```python
from build123d import *

# Parameters (mm, degrees)
BOSS_EXTRU_1_DEPTH      = 4
TROU_TARAUD_M42_D       = 3.3
TROU_TARAUD_M43_D       = 3.3
TROU_TARAUD_M43_DEPTH   = 15.5
TROU_TARAUD_M43_TIP     = 0.991420021
CONG_1_R                = 10
ENL_V_START             = -9
ENL_V_MAT_EXTRU_1_DEPTH = 10
CHANFREIN1_SIZE         = 1


with BuildPart() as part:
    # Esquisse1 → Boss.-Extru.1 (new body, symmetric)
    with BuildSketch(Plane.XY):
        with BuildLine():
            Line((-29, 0), (29, 0))
            Line((29, 0), (42.125962847, 19.175742472))
            ThreePointArc((42.125962847, 19.175742472), (42.080485732, 24.889573705), (36.705904774, 26.829629131))
            Line((36.705904774, 26.829629131), (0, 16.99431159))
            Line((0, 16.99431159), (-36.705904774, 26.829629131))
            ThreePointArc((-36.705904774, 26.829629131), (-42.080485732, 24.889573705), (-42.125962847, 19.175742472))
            Line((-42.125962847, 19.175742472), (-29, 0))
        make_face()
    extrude(amount=BOSS_EXTRU_1_DEPTH, both=True)

    # Trou taraudé M42 (through all)
    with Locations(Plane.XY.offset(4)):
        with Locations((-38, 22), (38, 22), (-33, 16), (33, 16)):
            Hole(TROU_TARAUD_M42_D / 2)

    # Trou taraudé M43
    with Locations(Plane(origin=(0, 0, 0), x_dir=(-1, 0, 0), z_dir=(0, -1, 0))):
        with Locations((20, 0), (-20, 0), (0, -0.5)):
            Hole(TROU_TARAUD_M43_D / 2, depth=TROU_TARAUD_M43_DEPTH)
            with Locations((0, 0, -(TROU_TARAUD_M43_DEPTH + TROU_TARAUD_M43_TIP / 2))):  # 118° drill point
                Cone(0, TROU_TARAUD_M43_D / 2, TROU_TARAUD_M43_TIP, mode=Mode.SUBTRACT)

    # Congé1
    cong_1_edges = [part.edges().sort_by_distance(p)[0] for p in [
        (0, 16.99431159, 0),
    ]]
    fillet(cong_1_edges, radius=CONG_1_R)

    # Esquisse8 → Enlèv. mat.-Extru.1 (cut)
    with BuildSketch(Plane.XY.offset(4).offset(ENL_V_START)):
        with BuildLine():
            Line((-3, 10.703460795), (-3, 10.5))
            ThreePointArc((-3, 10.5), (-3.732233047, 8.732233047), (-5.5, 8))
            Line((-5.5, 8), (-22.251200511, 8))
            ThreePointArc((-22.251200511, 8), (-23.417321879, 8.288629168), (-24.314181934, 9.087871236))
            Line((-24.314181934, 9.087871236), (-28.247222943, 14.833657842))
            ThreePointArc((-28.247222943, 14.833657842), (-28.224484386, 17.690573459), (-25.537193907, 18.660601172))
            Line((-25.537193907, 18.660601172), (-4.852952387, 13.118275361))
            ThreePointArc((-4.852952387, 13.118275361), (-3.516616649, 12.225364367), (-3, 10.703460795))
        make_face()
    enl_v_mat_extru_1 = extrude(amount=ENL_V_MAT_EXTRU_1_DEPTH, mode=Mode.SUBTRACT)

    # Symétrie1: Enlèv. mat.-Extru.1 across plane
    add(enl_v_mat_extru_1.mirror(Plane(origin=(0, 0, 0), x_dir=(0, 0, 1), z_dir=(1, 0, 0))), mode=Mode.SUBTRACT)

    # Chanfrein1
    chanfrein1_edges = [part.edges().sort_by_distance(p)[0] for p in [
        (-35.562981423, 9.587871236, -4),
        (-42.080485732, 24.889573705, 4),
        (-42.080485732, 24.889573705, -4),
        (-19.647047613, 22.258722131, -4),
        (-35.562981423, 9.587871236, 4),
        (35.562981423, 9.587871236, 4),
        (42.080485732, 24.889573705, 4),
        (-19.647047613, 22.258722131, 4),
        (19.647047613, 22.258722131, -4),
        (19.647047613, 22.258722131, 4),
        (0, 17.347073394, -4),
        (0, 17.347073394, 4),
        (42.080485732, 24.889573705, -4),
        (35.562981423, 9.587871236, -4),
    ]]
    chamfer(chanfrein1_edges, length=CHANFREIN1_SIZE)


solid = part.part
```
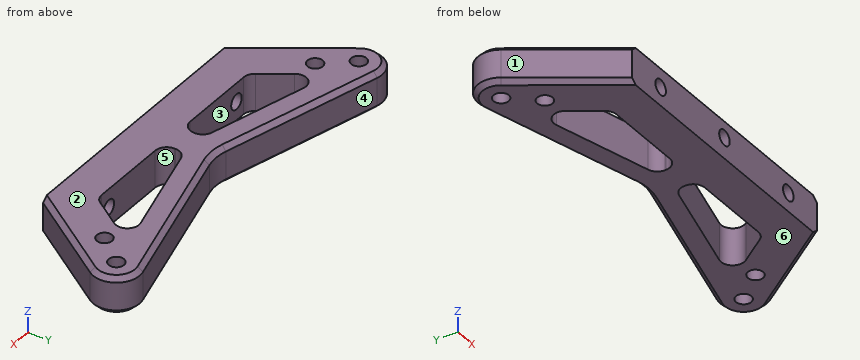
Geometry check sheet. Reference: the model listing, model coordinates, mm. Face numbers are marked on the shaded views. A direction names the side the tool comes from. Give positions to 0.01 mm unless a question says otherwise; leave off trailing zeros. Order: outer loops, then holes, each group sorted by start corner. A loop starts at its lowest first (then second) coordinate and runs counter-clockwise, first axis right, second up. Notation, with made-up numbers: (-0.75, -37.75) -> (39.25, -37.75) arc R18 cw to (39.25, -22.75) -> close; hole circle Ø8 at (36.5, -25.5). An arc over 180 degrees is marked (long way). Write each question's results on one line, items separated by ' | '. Start each with the question number.
(1) Sectioned sample at C-C (x = -20). Enter the section's corners in (y, z).
(2) Sectioned sample at D-D (x = 23.5). Enter the section's corners in (y, z).
(3) Scan lines: line 1 (Z direction, x = 20, y = 1.5); line 2 (X direction, y = 2.5, z = -0.75); line 3 (Y direction, x = -2.5, z = -2). Record each from-to range of solid material in increasing order.
(4) Sectioned sample at A-A (x = -33). Enter the section's corners in (y, z).
(5) Sectioned sample at B-B (y = 22). Enter the section's corners in (x, z).
(6) Access from +Z, -Z, +X, -X, +Y, -Y to the whole of each face (thin tool, end or side, straight path). Record for the marked faces 4, 5 and 6.
(7) Mould release check, pull along X, two halves, no side actions. Record for the marked faces 1, 2 and 3: pulls with the +X half, pulls with the -X half, needs draft (parallel to the pull), parting line crosses it, or undercut.
(8) Gauge pin test, flat ends, axial feed: P1, Ø3, axis at y = 10, z = 3, coming from the -X side; P2, Ø1, axis at x = -4.5, z = -2, coming from the +Y side; P3, Ø2.5, axis at x = 18, z = 1, coming from the +Y side. Record the tip position at first contact, or that the pin passes through.
Answer below:
1) outline: (0, -4) -> (8, -4) -> (8, -1.65) -> (0, -1.65) -> close; (0, 1.65) -> (8, 1.65) -> (8, 4) -> (0, 4) -> close; (17.18, -4) -> (21.32, -4) -> (22.35, -3) -> (22.35, 3) -> (21.32, 4) -> (17.18, 4) -> close
2) outline: (0, -4) -> (8.33, -4) -> (8.33, 4) -> (0, 4) -> close; (18.11, -4) -> (22.26, -4) -> (23.29, -3) -> (23.29, 3) -> (22.26, 4) -> (18.11, 4) -> close
3) line 1: -4 to -1.65, 1.65 to 4 | line 2: -30.71 to -21.47, -18.53 to -1.08, 1.08 to 18.53, 21.47 to 30.71 | line 3: 0 to 17.66
4) outline: (5.84, -3) -> (7.61, -4) -> (14.35, -4) -> (14.35, 4) -> (7.61, 4) -> (5.84, 3) -> close; (17.65, -4) -> (24.8, -4) -> (25.84, -3) -> (25.84, 3) -> (24.8, 4) -> (17.65, 4) -> close
5) outline: (-43, -3) -> (-42, -4) -> (-39.65, -4) -> (-39.65, 4) -> (-42, 4) -> (-43, 3) -> close; (-36.35, -4) -> (-22.55, -4) -> (-18.68, -3) -> (-18.68, 3) -> (-22.55, 4) -> (-36.35, 4) -> close; (18.68, -3) -> (22.55, -4) -> (36.35, -4) -> (36.35, 4) -> (22.55, 4) -> (18.68, 3) -> close; (39.65, -4) -> (42, -4) -> (43, -3) -> (43, 3) -> (42, 4) -> (39.65, 4) -> close
6) face 4: +Z, -Z, +Y | face 5: +Z, -Z | face 6: -Z, +X, -X, +Y, -Y
7) face 1: pulls with the -X half | face 2: needs draft | face 3: undercut
8) P1: x = -36.87 | P2: y = 18.33 | P3: y = 22.15
